```python
from build123d import *

# Parameters (mm, degrees)
F0_R     = 10.7
F1_DEPTH = 2
F2_R     = 3.75
F3_DEPTH = 11


with BuildPart() as f1:
    # F0 (on Top) → F1 (new body)
    with BuildSketch(Plane.XY):
        Circle(F0_R)
    extrude(amount=F1_DEPTH)

    # F2 (on Top) → F3 (join)
    with BuildSketch(Plane.XY):
        Circle(F2_R)
    extrude(amount=-F3_DEPTH)

    # F4 (on Front) → F5 (revolve)
    with BuildSketch(Plane.XZ):
        with BuildLine():
            Line((-4.3987915084, 0), (-10.7987915084, 0))
            Line((-10.7987915084, 0), (-10.7987915084, -11))
            Line((-10.7987915084, -11), (-10.3134103119, -11))
            ThreePointArc((-10.3134103119, -11), (-8.3948121612, -4.9414926276), (-4.3987915084, 0))
        make_face()
    revolve(axis=Axis((0, 0, -4.4246494012), (0, 0, -1)))


solid = f1.part
```
The listing builds one solid part. Answer for the finished solid, in the listing's coordinates (mm). A direction names the side the tool comes from. Coordinates: 2 decimals unless noted, no trailing zeros. Return JSON: item names as keys, results as strings. Group by question number.
1. Which of the six approach directions +Z, -Z, +X, -X, +Y, -Y give full straight-line access (tool end or side, diameter ignored) to faces 1 (the flat face through (0, 0, -11)), 2 (the cylindrical face through (-2.32, -10.446, 0.986))?
2. Given pin 1 (1.5 mm diameter, centred on x = -6, z = -1, fed in from +Y); pin 2 (1 mm diameter, centred on y = 8.5, z = -5, fed in from +X); pin 3 (1.5 mm diameter, centred on x = -4.5, z = -9, fed in from -Y), each flat-ended and moving along its own axis, determine where each tip first touches the part or whether it passes through.
3. Straight lines are drawn through the part: L1, parallel to X at y = -3, z = -4.5; L2, parallel to Y at x = 0, z = -10; L3, parallel to X at y = -2, z = -4. For each, find the intervals that lie inside material, in ascending order.
4. A cutting plane is placed at A-A, the plane z = -2. Give the number of separate pieces and of enclosed holes in the cut face, plus the area to 3 significant figures.
5. Determine the mould class of faces 3 (the flat face through (4, 1, 0)), 4 (the cylindrical face through (-4.98, -9.58, -5.58)), 5 (the cylindrical face through (-3.746, 0.165, -5.423)), 6 (the flat face through (0, 0, 2)) for opening direction X: released by +X, released by -X, zero draft, split by the parting line, or undercut.
Ans:
{
 "1": {"face 1": "-Z, +X, -X, +Y, -Y", "face 2": "+Z"},
 "2": {"pin 1": "y = 9.44", "pin 2": "x = 7.25", "pin 3": "y = -10.13"},
 "3": {"L1": "-10.37 to -7.58, -2.25 to 2.25, 7.58 to 10.37", "L2": "-10.8 to -10.16, -3.75 to 3.75, 10.16 to 10.8", "L3": "-10.61 to -7.59, -3.17 to 3.17, 7.59 to 10.61"},
 "4": {"separate pieces": "2", "enclosed holes": "1", "area": "282 mm²"},
 "5": {"face 3": "undercut", "face 4": "split by the parting line", "face 5": "undercut", "face 6": "zero draft"}
}
